Work out the finished part from the listing and answer in its coordinate system (mm). Face numbers are marked on the shaded views. A direction names the side the tool comes from. Round coordinates to 2 decimals unless told otherwise and drop trailing zeros. Order: outer loops, then holes, each group sorted by start corner. A loop starts at its lowest first (then second) coordinate and runs counter-clockwise, first axis right, second up. Notation, with made-up numbers: (65, 85.25) - (106, 85.25) arc R30 ccw to (106, 121.25) - close; hole circle Ø11 at (-3, -3). An arc over 180 degrees is marked (long way). Answer in a Markdown table with one row per item.
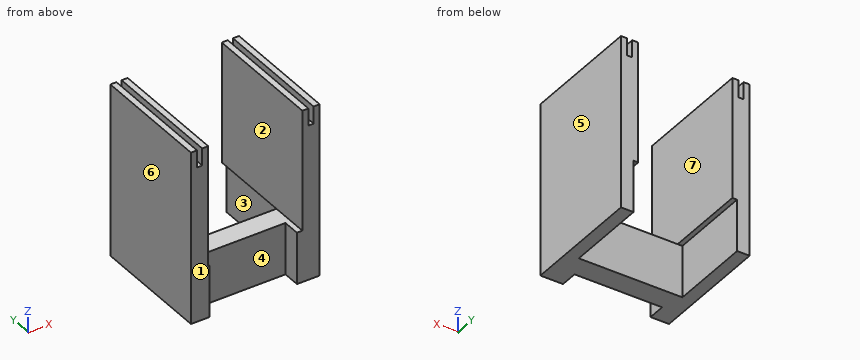
from build123d import *

# Parameters (mm, degrees)
SKETCH1_W           = 74.5
SKETCH1_H           = 100
BOSS_EXTRUDE1_DEPTH = 70
SKETCH3_W           = 54.5
SKETCH3_H           = 70
CUT_EXTRUDE1_DEPTH  = 144.004370563
SKETCH5_W           = 60
SKETCH5_H           = 30
CUT_EXTRUDE2_DEPTH  = 47.5
SKETCH6_W           = 3
SKETCH6_H           = 10
CUT_EXTRUDE3_DEPTH  = 144.004370563
SKETCH7_W           = 3
SKETCH7_H           = 10
CUT_EXTRUDE4_DEPTH  = 144.004370563
SKETCH10_W          = 50.670772636
SKETCH10_H          = 10
CUT_EXTRUDE5_DEPTH  = 144.004370563


with BuildPart() as part:
    # Sketch1 → Boss-Extrude1 (new body)
    with BuildSketch(Plane(origin=(0, 0, 0), x_dir=(1, 0, 0), z_dir=(0, 1, 0))):
        with Locations((37.25, 50)):
            Rectangle(SKETCH1_W, SKETCH1_H)
    extrude(amount=BOSS_EXTRUDE1_DEPTH)

    # Sketch3 → Cut-Extrude1 (cut, through all)
    with BuildSketch(Plane(origin=(0, 70, 0), x_dir=(1, 0, 0), z_dir=(0, 1, 0))):
        with Locations((37.25, 35)):
            Rectangle(SKETCH3_W, SKETCH3_H)
    extrude(amount=-CUT_EXTRUDE1_DEPTH, mode=Mode.SUBTRACT)

    # Sketch5 → Cut-Extrude2 (cut)
    with BuildSketch(Plane(origin=(0, 70, 0), x_dir=(1, 0, 0), z_dir=(0, 1, 0))):
        with Locations((37.25, 85)):
            Rectangle(SKETCH5_W, SKETCH5_H)
    extrude(amount=-CUT_EXTRUDE2_DEPTH, mode=Mode.SUBTRACT)

    # Sketch6 → Cut-Extrude3 (cut, through all)
    with BuildSketch(Plane(origin=(0, 70, 0), x_dir=(1, 0, 0), z_dir=(0, 1, 0))):
        with Locations((69.5, 5)):
            Rectangle(SKETCH6_W, SKETCH6_H)
    extrude(amount=-CUT_EXTRUDE3_DEPTH, mode=Mode.SUBTRACT)

    # Sketch7 → Cut-Extrude4 (cut, through all)
    with BuildSketch(Plane(origin=(0, 70, 0), x_dir=(1, 0, 0), z_dir=(0, 1, 0))):
        with Locations((5, 5)):
            Rectangle(SKETCH7_W, SKETCH7_H)
    extrude(amount=-CUT_EXTRUDE4_DEPTH, mode=Mode.SUBTRACT)

    # Sketch10 → Cut-Extrude5 (cut, through all)
    with BuildSketch(Plane(origin=(0, 0, -100), x_dir=(-1, 0, 0), z_dir=(0, 0, -1))):
        with Locations((-36.030583725, 5)):
            Rectangle(SKETCH10_W, SKETCH10_H)
    extrude(amount=-CUT_EXTRUDE5_DEPTH, mode=Mode.SUBTRACT)


solid = part.part
1) Find section D-D, the plane z = -90. Give the vertices of the cut face in (x, y), then the cut area to 3 significant figures.
Filled in:
| item | result |
|---|---|
| outline | (0, 0) - (10.7, 0) - (10.7, 10) - (61.37, 10) - (61.37, 0) - (74.5, 0) - (74.5, 70) - (67.25, 70) - (67.25, 22.5) - (7.25, 22.5) - (7.25, 70) - (0, 70) - close |
| area | 1,860 mm^2 |
2) Each of these flat-tipped pins is pushed along its axis until it touches: pin 1 (5 mm diameter, centred on x = 13.5, z = -33, fed in from +Y); pin 2 (15 mm diameter, centred on x = 36, z = -91, fed in from +Y); pin 3 (0.8 mm diameter, centred on x = 65.5, y = 43, fed in from -Z); pin 4 (24 mm diameter, centred on x = 46, z = -90.5, fed in from -Y). Where does it stop, or does it pass through?
Filled in:
| item | result |
|---|---|
| pin 1 | passes through |
| pin 2 | stops at y = 22.5 |
| pin 3 | stops at z = -70 |
| pin 4 | stops at y = 10 |
3) Find section C-C, the plane y = 12.5. Give the vertices of the cut face in (x, z).
Filled in:
| item | result |
|---|---|
| outline | (0, -100) - (74.5, -100) - (74.5, 0) - (71, 0) - (71, -10) - (68, -10) - (68, 0) - (64.5, 0) - (64.5, -70) - (10, -70) - (10, 0) - (6.5, 0) - (6.5, -10) - (3.5, -10) - (3.5, 0) - (0, 0) - close |
4) The mould has two halves that part along X. Classify the marked faces 5, 6 and 7: released by +X, released by -X, zero draft, split by the parting line, or undercut.
Filled in:
| item | result |
|---|---|
| face 5 | released by +X |
| face 6 | released by -X |
| face 7 | undercut |
5) Find section B-B, the plane y = 65. Give the vertices of the cut face in (x, z).
Filled in:
| item | result |
|---|---|
| outline | (0, -100) - (7.25, -100) - (7.25, -70) - (10, -70) - (10, 0) - (6.5, 0) - (6.5, -10) - (3.5, -10) - (3.5, 0) - (0, 0) - close; (64.5, -70) - (67.25, -70) - (67.25, -100) - (74.5, -100) - (74.5, 0) - (71, 0) - (71, -10) - (68, -10) - (68, 0) - (64.5, 0) - close |
6) Find the intervals of material crossed by probe 1 along X at (y, z) = (27.5, -78); probe 2 along X at (y, z) = (20, -52); probe 3 along Z at (x, y) = (20.5, 16.5), in increasing order. Write a range as from..to.
Filled in:
| item | result |
|---|---|
| probe 1 | x = 0..7.25, 67.25..74.5 |
| probe 2 | x = 0..10, 64.5..74.5 |
| probe 3 | z = -100..-70 |
7) Find section A-A, the plane z = -27. Give the vertices of the cut face in (x, y), then the cut area to 3 significant figures.
Filled in:
| item | result |
|---|---|
| outline | (0, 0) - (10, 0) - (10, 70) - (0, 70) - close; (64.5, 0) - (74.5, 0) - (74.5, 70) - (64.5, 70) - close |
| area | 1,400 mm^2 |
8) Which of the six approach directions +Z, -Z, +X, -X, +Y, -Y give full straight-line access (tool end or side, diameter ignored) to the marked faces 1, 2, 3 and 4?
Filled in:
| item | result |
|---|---|
| face 1 | +Z, -Z, +X, -X, -Y |
| face 2 | +Z, +Y, -Y |
| face 3 | -Z, +Y |
| face 4 | +Z, -Z, -Y |
